For this review, use the dimensioned drawing (mm, ordinates from the lowest corner) and the shaded views. A direction names the side the tool comes from. Round coordinates to 2 decimals unless told otherwise and drop trailing zeros. Order: outer loops, then holes, each group sorted by start corner. A loop starts at its lowest first (then second) coordinate and runs counter-clockwise, first axis right, second up. Notation, with made-up numbers: (-27, 45) - (-10, 45) arc R23 cw to (-10, 56) - close; hole circle Ø7 at (-2.75, -29). An arc over 180 degrees is marked (long way). Write each question's results on one line, items separated by ' | '. Start each with the question number.
(1) Take a section at A-A, the plane x = 5. Give the boundary of the cut face in (y, z).
(2) For L1, parallel to Z at x = 5, y = 5.8; L2, parallel to Z at x = 8, y = 6.5; L3, parallel to X at y = 5.95, z = 29.3, list the stretches that pass through material, from the lowest coordinate up. Write a range as from..to.
(3) For the marked faces 1 and 2, list the 3-axis set-ups (+Z, -Z, +X, -X, +Y, -Y) from which the entire face can be reached by the end or side of a thin tool; tool diameter is ignored.
(4) Take a section at D-D, the plane x = 2. Give the boundary of the cut face in (y, z).
(5) Insertion check: pin 1 Ø4 at (y, z) = (4.5, 17.5) entering from +X; pin 2 Ø3 at (y, z) = (7.5, 20.5) entering from -X; pin 3 Ø6 at (y, z) = (2, 26) entering from -X. Each pin has a flat end and moves straight along its axis. Give the tip position at first contact, or say it passes through.
(6) Take a section at B-B, the plane y = 5. Give the boundary of the cut face in (x, z).
(7) Take a section at C-C, the plane z = 29.3. Give the boundary of the cut face in (x, y).
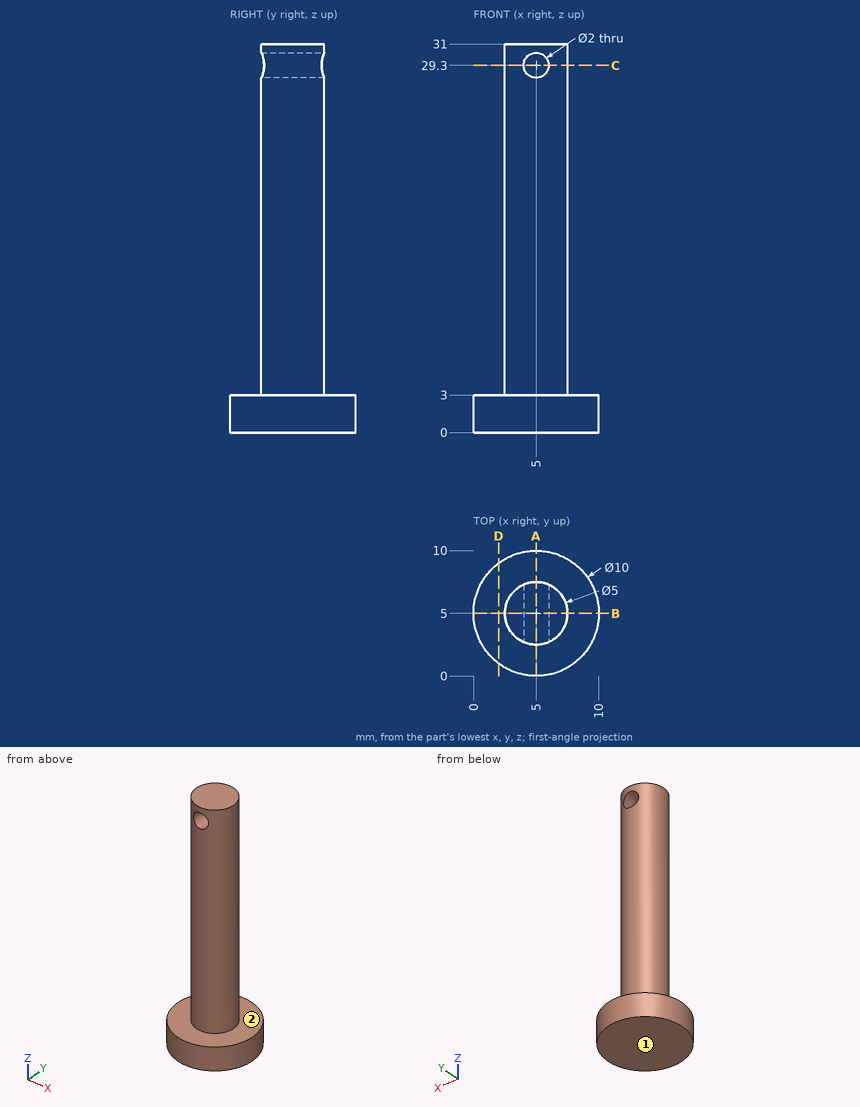
Results below:
1) outline: (0, 0) - (10, 0) - (10, 3) - (7.5, 3) - (7.5, 28.3) - (2.5, 28.3) - (2.5, 3) - (0, 3) - close; (2.5, 30.3) - (7.5, 30.3) - (7.5, 31) - (2.5, 31) - close
2) L1: z = 0..28.3, 30.3..31 | L2: z = 0..3 | L3: x = 2.69..4, 6..7.31
3) face 1: -Z, +X, -X, +Y, -Y | face 2: +Z
4) outline: (1, 0) - (9, 0) - (9, 3) - (1, 3) - close
5) pin 1: stops at x = 7.5 | pin 2: stops at x = 2.71 | pin 3: stops at x = 2.5
6) outline: (0, 0) - (10, 0) - (10, 3) - (7.5, 3) - (7.5, 31) - (2.5, 31) - (2.5, 3) - (0, 3) - close; hole circle Ø2 at (5, 29.3)
7) outline: (4, 2.71) - (4, 7.29) arc R2.5 ccw to start; (6, 2.71) arc R2.5 ccw to (6, 7.29) - close
